Drawing for the job (mm, zero at the part's lowest x, y, z). A direction names the side the tool comes from. Coordinates: 2 decimals unless noted, no trailing zeros. Write each loop counter-clockwise with the first axis right and the second up, starting at its lowest first coordinate (ties: lowest second). Pieces come first, ordered by that corner, then holes. Notation, with made-up numbers: (-32, 37.25) -> (-14, 37.25) arc R13 ccw to (-14, 50.25) -> close; hole circle Ø5 at (7.25, 61.5). An arc over 180 degrees is marked (long way). Answer as CSV lines item,"result".
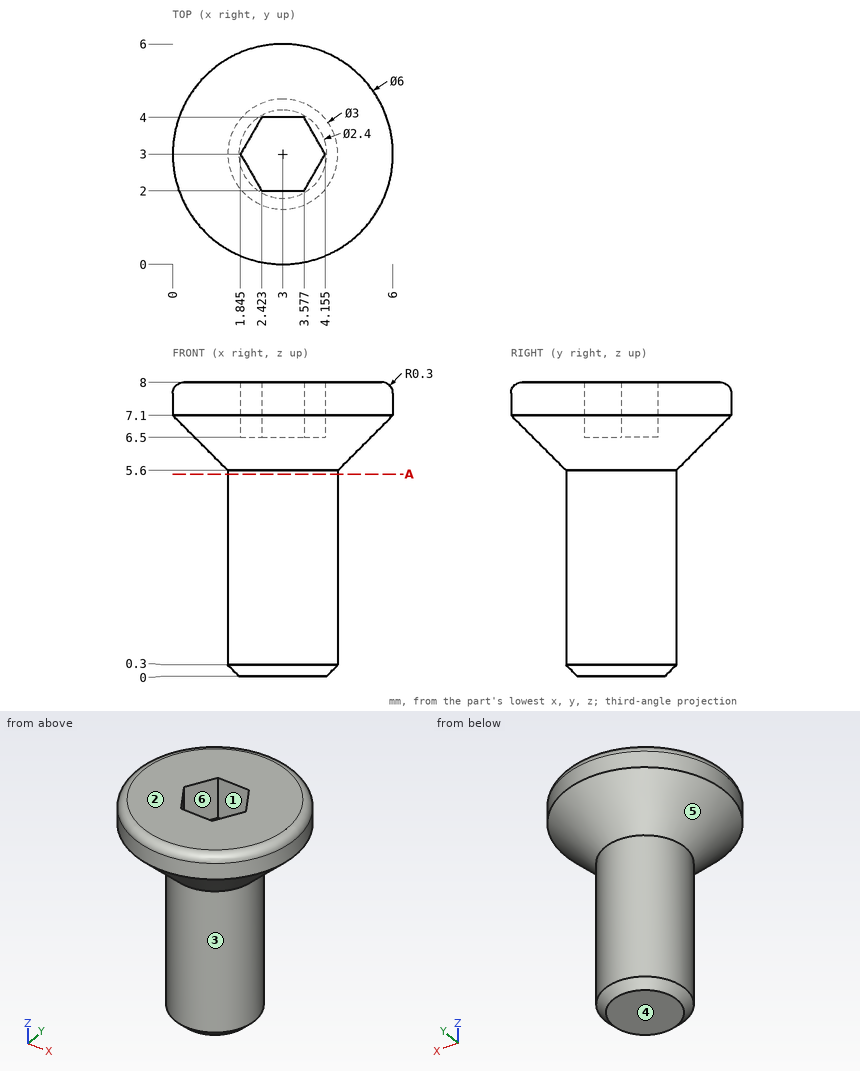
Item 1: Two-plate mould, pull along X, no slides. Class the marked faces 4, 5 and 6: pulls with the +X half, pulls with the -X half, needs draft (parallel to the pull), parting line crosses it, or undercut.
Answer below:
face 4,"needs draft"
face 5,"parting line crosses it"
face 6,"undercut"
Item 2: 3-axis set-ups, long thin cutter, end or side, ignore diameter. For the marked faces 1, 2 and 3: which of +Z, -Z, +X, -X, +Y, -Y reach the whole face in a straight line?
Answer below:
face 1,"+Z"
face 2,"+Z, +X, -X, +Y, -Y"
face 3,"-Z"
Item 3: Saw through at A-A on z = 5.5. Give the cut face in (x, y).
Answer below:
outline,"circle Ø3 at (3, 3)"
Item 4: Flat gauge pins, fed straight in: pin 1 (3 mm diameter, centred on y = 2.5, z = 1, fed in from +X); pin 2 (0.6 mm diameter, centred on x = 2.5, z = 7.5, fed in from +Y); pin 3 (1.3 mm diameter, centred on x = 3, z = 7, fed in from -Y); pin 4 (0.6 mm diameter, centred on x = 2.5, y = 3, fed in from +Z). Where does each tip first touch, or does it go through?
Answer below:
pin 1,"stops at x = 4.5"
pin 2,"stops at y = 5.99"
pin 3,"stops at y = 0"
pin 4,"stops at z = 6.5"
Item 5: Wall check: line 1 (Z direction, x = 3.25, y = 3.25); line 2 (X direction, y = 3.75, z = 5.75); line 3 (Y direction, x = 2.5, z = 2.5) (1 decimal). Give the ranges that are in metal, low to high. Write a range as from..to.
Answer below:
line 1,"z = 0..6.5"
line 2,"x = 1.53..4.47"
line 3,"y = 1.6..4.4"
